Build history of the part. All positions in model axes, mm. A direction names the side the tool comes from. Round coordinates to 2 decimals unless told otherwise and drop trailing zeros. Write each loop counter-clockwise with the first axis right and the second up, starting at its lowest first coordinate (ties: lowest second). Pieces come first, ordered by that corner, then holes.
1) Pull direction X, two halves, no side cores. Call faces 1 (the flat face through (6.1, 5, 1.6)), 2 (the cylindrical face through (7.43, 4.95, 1.58)), 3 (the flat face through (-4, 0, 3.2)): +X half, -X half, draft (parallel to the pull), parting line (faces both ways), or undercut.
2) Wall check: probe 1 along Y at (x, z) = (7, 0.6); probe 2 along Y at (x, z) = (-7.25, 1.8). Give the ranges that are in metal, low to high.
3) Saw through at B-B (x = 4.25). Write the cut outline in (y, z), plus the area to 3 significant figures.
4) Saw through at A-A (y = -3.25). Write the cut outline in (x, z), plus the area to 3 significant figures.
5) Flat gauge pin, fed straight in: pin 1 (1.5 mm diameter, centred on y = 0, z = 2, fed in from +X). Where does the tip first touch, or does it go through?
6) Which spindle directions (+Z, -Z, +X, -X, +Y, -Y) get a long thin tool onto all of the face, cutting with end or side? Do faces 4 (the flat face through (7.562, -2.282, 1.623)), 5 (the flat face through (-0.77, -7.83, 1.62)), 6 (the flat face through (-6.94, 3.71, 1.62)), 7 (the flat face through (0.77, 7.83, 1.62)). Say none if no direction does.
from build123d import *

# Parameters (mm, degrees)
SKETCH1_R           = 8.926200703
BOSS_EXTRUDE1_DEPTH = 3.2004
CUT_EXTRUDE1_DEPTH  = 3.2004


with BuildPart() as part:
    # Sketch1 → Boss-Extrude1 (new body)
    with BuildSketch(Plane.XY):
        Circle(SKETCH1_R)
        Polygon((0, 3.048), (-0.315924789, 2.500802214), (-0.758006776, 2.952241475), (-0.927923651, 2.343667613), (-1.468385199, 2.670982761), (-1.481617658, 2.039271757), (-2.086499579, 2.221896376), (-1.942216178, 1.606740957), (-2.573511517, 1.633200071), (-2.280778112, 1.073252713), (-2.898820262, 0.941883799), (-2.47603037, 0.472328054), (-3.041985468, 0.191385504), (-2.515704533, -0.158274714), (-2.99401154, -0.571138247), (-2.397307729, -0.778932499), (-2.757912856, -1.297775281), (-2.128279263, -1.350647091), (-2.348524364, -1.942868321), (-1.725523184, -1.837495558), (-1.791569449, -2.465883799), (-1.214346137, -2.208887422), (-1.122043637, -2.833958729), (-0.626867256, -2.441486766), (-0.382015696, -3.02396561), (0, -2.520678517), (0.382015696, -3.02396561), (0.626867256, -2.441486766), (1.122043637, -2.833958729), (1.214346137, -2.208887422), (1.791569449, -2.465883799), (1.725523184, -1.837495558), (2.348524364, -1.942868321), (2.128279263, -1.350647091), (2.757912856, -1.297775281), (2.397307729, -0.778932499), (2.99401154, -0.571138247), (2.515704533, -0.158274714), (3.041985468, 0.191385504), (2.47603037, 0.472328054), (2.898820262, 0.941883799), (2.280778112, 1.073252713), (2.573511517, 1.633200071), (1.942216178, 1.606740957), (2.086499579, 2.221896376), (1.481617658, 2.039271757), (1.468385199, 2.670982761), (0.927923651, 2.343667613), (0.758006776, 2.952241475), (0.315924789, 2.500802214), align=None, mode=Mode.SUBTRACT)
    extrude(amount=BOSS_EXTRUDE1_DEPTH)

    # Sketch2 → Cut-Extrude1 (cut)
    with BuildSketch(Plane.XY.offset(3.2004)):
        with BuildLine():
            Line((-1.255122678, 8.837518093), (-0.301897322, 6.853917937))
            ThreePointArc((-0.301897322, 6.853917937), (0, 6.664048588), (0.301897322, 6.853917937))
            Line((0.301897322, 6.853917937), (1.255122678, 8.837518093))
            ThreePointArc((1.255122678, 8.837518093), (0, 8.926200703), (-1.255122678, 8.837518093))
        make_face()
        with BuildLine():
            Line((2.901797598, 6.216663396), (4.54155391, 7.68448743))
            ThreePointArc((4.54155391, 7.68448743), (3.415909123, 8.246734132), (2.222389605, 8.645116739))
            Line((2.222389605, 8.645116739), (2.343964085, 6.447725603))
            ThreePointArc((2.343964085, 6.447725603), (2.550220987, 6.156778094), (2.901797598, 6.216663396))
        make_face()
        with BuildLine():
            Line((5.059925495, 4.632978207), (7.136574729, 5.361563216))
            ThreePointArc((7.136574729, 5.361563216), (6.311777047, 6.311777047), (5.361563216, 7.136574729))
            Line((5.361563216, 7.136574729), (4.632978207, 5.059925495))
            ThreePointArc((4.632978207, 5.059925495), (4.712193947, 4.712193947), (5.059925495, 4.632978207))
        make_face()
        with BuildLine():
            Line((6.447725603, 2.343964085), (8.645116739, 2.222389605))
            ThreePointArc((8.645116739, 2.222389605), (8.246734132, 3.415909123), (7.68448743, 4.54155391))
            Line((7.68448743, 4.54155391), (6.216663396, 2.901797598))
            ThreePointArc((6.216663396, 2.901797598), (6.156778094, 2.550220987), (6.447725603, 2.343964085))
        make_face()
        with BuildLine():
            Line((6.853917937, -0.301897322), (8.837518093, -1.255122678))
            ThreePointArc((8.837518093, -1.255122678), (8.926200703, 0), (8.837518093, 1.255122678))
            Line((8.837518093, 1.255122678), (6.853917937, 0.301897322))
            ThreePointArc((6.853917937, 0.301897322), (6.664048588, 0), (6.853917937, -0.301897322))
        make_face()
        with BuildLine():
            Line((6.216663396, -2.901797598), (7.68448743, -4.54155391))
            ThreePointArc((7.68448743, -4.54155391), (8.246734132, -3.415909123), (8.645116739, -2.222389605))
            Line((8.645116739, -2.222389605), (6.447725603, -2.343964085))
            ThreePointArc((6.447725603, -2.343964085), (6.156778094, -2.550220987), (6.216663396, -2.901797598))
        make_face()
        with BuildLine():
            Line((4.632978207, -5.059925495), (5.361563216, -7.136574729))
            ThreePointArc((5.361563216, -7.136574729), (6.311777047, -6.311777047), (7.136574729, -5.361563216))
            Line((7.136574729, -5.361563216), (5.059925495, -4.632978207))
            ThreePointArc((5.059925495, -4.632978207), (4.712193947, -4.712193947), (4.632978207, -5.059925495))
        make_face()
        with BuildLine():
            Line((2.343964085, -6.447725603), (2.222389605, -8.645116739))
            ThreePointArc((2.222389605, -8.645116739), (3.415909123, -8.246734132), (4.54155391, -7.68448743))
            Line((4.54155391, -7.68448743), (2.901797598, -6.216663396))
            ThreePointArc((2.901797598, -6.216663396), (2.550220987, -6.156778094), (2.343964085, -6.447725603))
        make_face()
        with BuildLine():
            Line((-0.301897322, -6.853917937), (-1.255122678, -8.837518093))
            ThreePointArc((-1.255122678, -8.837518093), (0, -8.926200703), (1.255122678, -8.837518093))
            Line((1.255122678, -8.837518093), (0.301897322, -6.853917937))
            ThreePointArc((0.301897322, -6.853917937), (0, -6.664048588), (-0.301897322, -6.853917937))
        make_face()
        with BuildLine():
            Line((-2.901797598, -6.216663396), (-4.54155391, -7.68448743))
            ThreePointArc((-4.54155391, -7.68448743), (-3.415909123, -8.246734132), (-2.222389605, -8.645116739))
            Line((-2.222389605, -8.645116739), (-2.343964085, -6.447725603))
            ThreePointArc((-2.343964085, -6.447725603), (-2.550220987, -6.156778094), (-2.901797598, -6.216663396))
        make_face()
        with BuildLine():
            Line((-5.059925495, -4.632978207), (-7.136574729, -5.361563216))
            ThreePointArc((-7.136574729, -5.361563216), (-6.311777047, -6.311777047), (-5.361563216, -7.136574729))
            Line((-5.361563216, -7.136574729), (-4.632978207, -5.059925495))
            ThreePointArc((-4.632978207, -5.059925495), (-4.712193947, -4.712193947), (-5.059925495, -4.632978207))
        make_face()
        with BuildLine():
            Line((-6.447725603, -2.343964085), (-8.645116739, -2.222389605))
            ThreePointArc((-8.645116739, -2.222389605), (-8.246734132, -3.415909123), (-7.68448743, -4.54155391))
            Line((-7.68448743, -4.54155391), (-6.216663396, -2.901797598))
            ThreePointArc((-6.216663396, -2.901797598), (-6.156778094, -2.550220987), (-6.447725603, -2.343964085))
        make_face()
        with BuildLine():
            Line((-6.853917937, 0.301897322), (-8.837518093, 1.255122678))
            ThreePointArc((-8.837518093, 1.255122678), (-8.926200703, 0), (-8.837518093, -1.255122678))
            Line((-8.837518093, -1.255122678), (-6.853917937, -0.301897322))
            ThreePointArc((-6.853917937, -0.301897322), (-6.664048588, 0), (-6.853917937, 0.301897322))
        make_face()
        with BuildLine():
            Line((-6.216663396, 2.901797598), (-7.68448743, 4.54155391))
            ThreePointArc((-7.68448743, 4.54155391), (-8.246734132, 3.415909123), (-8.645116739, 2.222389605))
            Line((-8.645116739, 2.222389605), (-6.447725603, 2.343964085))
            ThreePointArc((-6.447725603, 2.343964085), (-6.156778094, 2.550220987), (-6.216663396, 2.901797598))
        make_face()
        with BuildLine():
            Line((-4.632978207, 5.059925495), (-5.361563216, 7.136574729))
            ThreePointArc((-5.361563216, 7.136574729), (-6.311777047, 6.311777047), (-7.136574729, 5.361563216))
            Line((-7.136574729, 5.361563216), (-5.059925495, 4.632978207))
            ThreePointArc((-5.059925495, 4.632978207), (-4.712193947, 4.712193947), (-4.632978207, 5.059925495))
        make_face()
        with BuildLine():
            Line((-2.343964085, 6.447725603), (-2.222389605, 8.645116739))
            ThreePointArc((-2.222389605, 8.645116739), (-3.415909123, 8.246734132), (-4.54155391, 7.68448743))
            Line((-4.54155391, 7.68448743), (-2.901797598, 6.216663396))
            ThreePointArc((-2.901797598, 6.216663396), (-2.550220987, 6.156778094), (-2.343964085, 6.447725603))
        make_face()
    extrude(amount=-CUT_EXTRUDE1_DEPTH, mode=Mode.SUBTRACT)


solid = part.part
Evaluation:
1. face 1: undercut
1. face 2: +X half
1. face 3: draft
2. probe 1: y = -5.31 to -3.78, -2.31 to -0.37, 0.37 to 2.31, 3.78 to 5.31
2. probe 2: y = -5.21 to -4.06, -2.3 to -0.49, 0.49 to 2.3, 4.06 to 5.21
3. outline: (-7.42, 0) - (7.42, 0) - (7.42, 3.2) - (-7.42, 3.2) - close
3. area: 47.5 mm2
4. outline: (-6.53, 0) - (6.53, 0) - (6.53, 3.2) - (-6.53, 3.2) - close
4. area: 41.8 mm2
5. pin 1: stops at x = 7.79
6. face 4: +Z, -Z, +X
6. face 5: +Z, -Z, -Y
6. face 6: +Z, -Z, -X
6. face 7: +Z, -Z, +Y
